Autodesk Inventor part; units mm, degrees
ref_plane "YZ Plane" through (0, 0, 0) normal (1, 0, 0) x (0, 1, 0)
ref_plane "XZ Plane" through (0, 0, 0) normal (0, 1, 0) x (-1, 0, 0)
ref_plane "XY Plane" through (0, 0, 0) normal (0, 0, 1) x (1, 0, 0)
sketch "Sketch1" plane through (0, 0, 0) normal (0, 1, 0) x (-1, 0, 0)
  circle A0 centre (0, 0) radius 17.5
  circle A1 centre (0, 0) radius 2.5
  dimension "d0" = 35
  dimension "d1" = 5
extrude "Extrusion1" add sketch "Sketch1" against normal blind 25
thicken "Thicken1" operation add thickness 1 both sides no extend neighbours yes toward (-0.9967573, 0, -0.0804666) faces at (-17.4433, -16.6667, -1.4082)
thicken "Thicken2" operation add thickness 1 both sides no extend neighbours yes toward (-0.9967573, 0, -0.0804666) faces at (-18.44, -16.6667, -1.4886)
properties part number "roller2 grp17"
The model under review builds one solid part; all positions refer to its coordinate system, in mm. Give positions to 0.01 mm unless a question says otherwise; leave off trailing zeros. Write each loop counter-clockwise with the first axis right and the second up, starting at its lowest first coordinate (ties: lowest second). Pieces come first, ordered by that corner, then holes. Notation, with made-up numbers: (27, -4) -> (50, -4) arc R9 ccw to (50, 9) -> close; hole circle Ø10 at (45, 34). An arc over 180 degrees is marked (long way). Put each result on its own line as item: value.
(1) We need section C-C, the plane y = -17.25. Give the boundary of the cut face in (x, z).
Results are:
outline: circle Ø39 at (0, 0); hole circle Ø5 at (0, 0)
(2) To check wall thickness, follow probe 1 along Z at (x, y) = (0, -18); probe 2 along Z at (x, y) = (2, -2.25). State the ranges of each line that lie inside material, in increasing order. Write a range as from..to.
Results are:
probe 1: -19.5..-2.5, 2.5..19.5
probe 2: -19.4..-1.5, 1.5..19.4
(3) The part is to be moulded in two halves that separate along Z. For faces 1 (the cylindrical face through (0.54, -12.32, -2.44)), 2 (the cylindrical face through (2.539, -12.325, 19.334)), 3 (the flat face through (0, -25, -4)), say which applies: pulls with the +Z half, pulls with the -Z half, needs draft (parallel to the pull), parting line crosses it, or undercut.
Results are:
face 1: undercut
face 2: parting line crosses it
face 3: needs draft
(4) We need section B-B, the plane z = 0. Give the boundary of the cut face in (x, y).
Results are:
outline: (-19.5, -25) -> (-2.5, -25) -> (-2.5, 0) -> (-19.5, 0) -> close; (2.5, -25) -> (19.5, -25) -> (19.5, 0) -> (2.5, 0) -> close
(5) For pin 1 Ø8 at (y, z) = (-18, -14.5) entering from +X; pin 2 Ø10 at (y, z) = (-19, -12) entering from -X; pin 3 Ø3 at (y, z) = (-17.5, -12) entering from -X; pin 4 Ø4 at (x, z) = (0, 0) entering from +Y, all flat-tipped, find the tip position at first contact; note any pin that passes through.
Results are:
pin 1: x = 16.43
pin 2: x = -18.2
pin 3: x = -16.43
pin 4: through
(6) We need section D-D, the plane z = -9.5. Give the boundary of the cut face in (x, y).
Results are:
outline: (-17.03, -25) -> (17.03, -25) -> (17.03, 0) -> (-17.03, 0) -> close
(7) We need section A-A, the plane x = 0. Give the boundary of the cut face in (y, z), and give its area (3 significant figures).
Results are:
outline: (-25, -19.5) -> (0, -19.5) -> (0, -2.5) -> (-25, -2.5) -> close; (-25, 2.5) -> (0, 2.5) -> (0, 19.5) -> (-25, 19.5) -> close
area: 850 mm²
